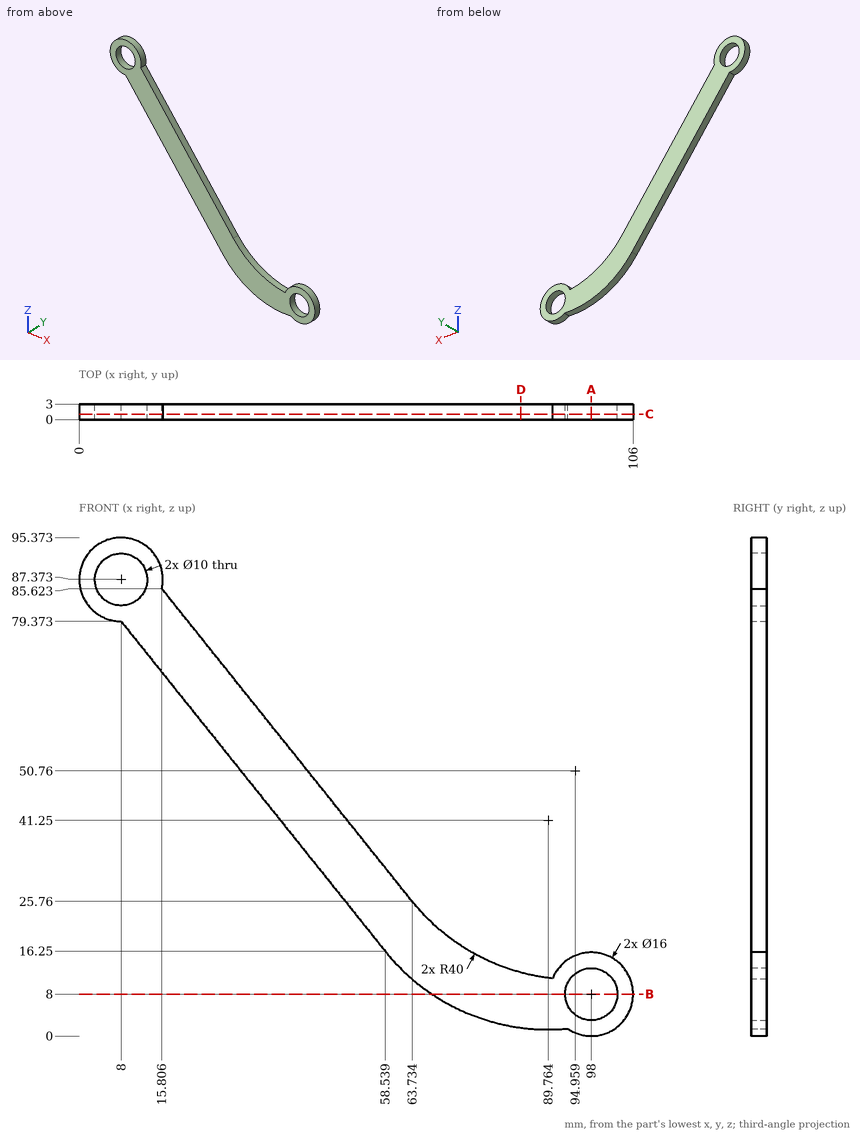
Source: three-view drawing plus pictorial views. Frame: mm from the lowest corner of the part. Round coordinates to 2 decimals unless told otherwise and drop trailing zeros. Loops run counter-clockwise (first coordinate to the right, second up) from the corner with the lowest first, then second, coordinate; pieces in that order, holes last. Notation, with made-up numbers: (-13, 6.25) - (-5, 6.25) arc R15 ccw to (-5, 28.25) - close; hole circle Ø8 at (52.5, 60.25). An arc over 180 degrees is marked (long way). Write item = value, one per line. Start each with the question number.
Item 1: Section query C-C on y = 1.05. Count the separate pieces of the cut face and the enclosed holes in it, plus the area to 3 significant figures.
Item 2: Section query D-D on x = 84.5. Output: boundary loops of the cut face in (y, z).
Item 3: Section query A-A on x = 98. Output: boundary loops of the cut face in (y, z).
Item 4: First-contact query: pin 1 Ø6 at (x, z) = (98, 8) entering from +Y. Flat tip, straight axial feed; report the tip coordinate or a pass-through.
Item 5: Material intervals for line 1 (Z direction, x = 8, y = 0.7) (1 decimal); line 2 (Z direction, x = 98, y = 0.9); line 3 (X direction, y = 0.55, z = 9) (1 decimal), sorted ascending.
Item 6: Section query B-B on z = 8. Output: boundary loops of the cut face in (x, y).
Results list:
q1.separate_pieces = 1
q1.enclosed_holes = 2
q1.area = 1,380 mm²
q2.outline = (0, 1.6) - (3, 1.6) - (3, 12.15) - (0, 12.15) - close
q3.outline = (0, 0) - (3, 0) - (3, 3) - (0, 3) - close; (0, 13) - (3, 13) - (3, 16) - (0, 16) - close
q4.pin_1 = through
q5.line_1 = 79.4 to 82.4, 92.4 to 95.4
q5.line_2 = 0 to 3, 13 to 16
q5.line_3 = 66.1 to 93.1, 102.9 to 105.9
q6.outline = (67.53, 0) - (93, 0) - (93, 3) - (67.53, 3) - close; (103, 0) - (106, 0) - (106, 3) - (103, 3) - close
